```python
from build123d import *

# Parameters (mm, degrees)
PAD_DEPTH         = 2
SKETCH001_W       = 2
SKETCH001_H       = 33.12
PAD001_DEPTH      = 34.6
PAD001_DEPTH_BACK = 2


with BuildPart() as part:
    # Sketch → Pad (new body)
    with BuildSketch(Plane.YZ):
        Polygon((-23.355, 0), (24.355, 0), (24.355, 13.665881), (-31.245, 13.665881), align=None)
    extrude(amount=PAD_DEPTH)

    # Sketch001 (on Face6 of Pad) → Pad001 (join, two sides)
    with BuildSketch(Plane.YZ.offset(2)) as pad001_sk:
        with Locations((0, 16.56)):
            Rectangle(SKETCH001_W, SKETCH001_H)
    extrude(amount=PAD001_DEPTH)
    extrude(pad001_sk.sketch, amount=-PAD001_DEPTH_BACK)


solid = part.part
```
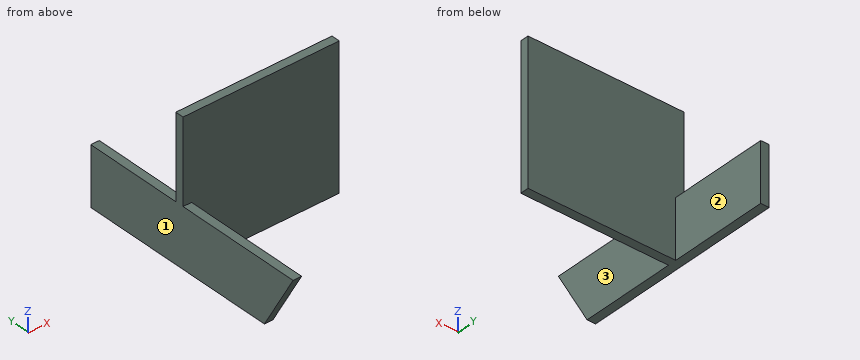
Here's how the part is built. I have some questions about the finished solid (model axes, mm). Face numbers are marked on the shaded views. A direction names the side the tool comes from. Coordinates: 2 decimals unless noted, no trailing zeros. Write each loop counter-clockwise with the first axis right and the second up, starting at its lowest first coordinate (ties: lowest second). Pieces come first, ordered by that corner, then holes. Notation, with made-up numbers: (30, -36.5) -> (65, -36.5) arc R22 ccw to (65, -22.5) -> close; hole circle Ø6 at (30.5, 50). An arc over 180 degrees is marked (long way). Use a Markdown table: item, result. Add a question column.
(1) I'm going to push flat-ended pins straight in: P1, Ø8, axis at y = -12, z = 3.5, coming from the +X side; P2, Ø12, axis at x = 28, z = 9, coming from the -Y side; P3, Ø1, axis at x = 1.5, y = 7.5, coming from the +Z side. Where does each tip first touch, or does it pass through?
(2) Please list where these lines run through material, in increasing order: line 1 (Y direction, x = 29, z = 25.5); line 2 (X direction, y = 15, z = 9).
(3) If we section it at D-D, the plane z = 11: Write out the boundary of the cut face in (x, y) (3 decimals).
(4) If we section it at A-A, the plane z = 4.5: Write out the boundary of the cut face in (x, y) (3 decimals).
(5) For the marked faces 1, 2 and 3, which set-ups out of +Z, -Z, +X, -X, +Y, -Y let a thin tool reach every point of the face, with its end or its side?
(6) If we section it at B-B, the plane y = 9.5: Write out the boundary of the cut face in (x, z).
(7) If we section it at C-C, the plane x = 11: Write out the boundary of the cut face in (y, z).
Outcome:
| question | item | result |
|---|---|---|
| 1 | P1 | stops at x = 2 |
| 1 | P2 | stops at y = -1 |
| 1 | P3 | stops at z = 13.67 |
| 2 | line 1 | y = -1 to 1 |
| 2 | line 2 | x = 0 to 2 |
| 3 | outline | (0, -29.706) -> (2, -29.706) -> (2, -1) -> (36.6, -1) -> (36.6, 1) -> (2, 1) -> (2, 24.355) -> (0, 24.355) -> close |
| 4 | outline | (0, -25.953) -> (2, -25.953) -> (2, -1) -> (36.6, -1) -> (36.6, 1) -> (2, 1) -> (2, 24.355) -> (0, 24.355) -> close |
| 5 | face 1 | +Z, -Z, -X, +Y, -Y |
| 5 | face 2 | +Z, -Z, +X, +Y |
| 5 | face 3 | +Z, -Z, +X, -Y |
| 6 | outline | (0, 0) -> (2, 0) -> (2, 13.67) -> (0, 13.67) -> close |
| 7 | outline | (-1, 0) -> (1, 0) -> (1, 33.12) -> (-1, 33.12) -> close |
